Here's the drawing with two shaded views (mm, measured from the low corner). I have some questions. A direction names the side the tool comes from. Coordinates: 2 decimals unless noted, no trailing zeros. Loops run counter-clockwise (first coordinate to the right, second up) from the corner with the lowest first, then second, coordinate; pieces in that order, holes last. Notation, with made-up numbers: (74.5, 47.25) -> (133.5, 47.25) arc R20 cw to (133.5, 75.25) -> close; hole circle Ø5 at (44.25, -4.5). An arc over 180 degrees is marked (long way). Use CSV: the item, a comma, the result in double quotes. Start each with the question number.
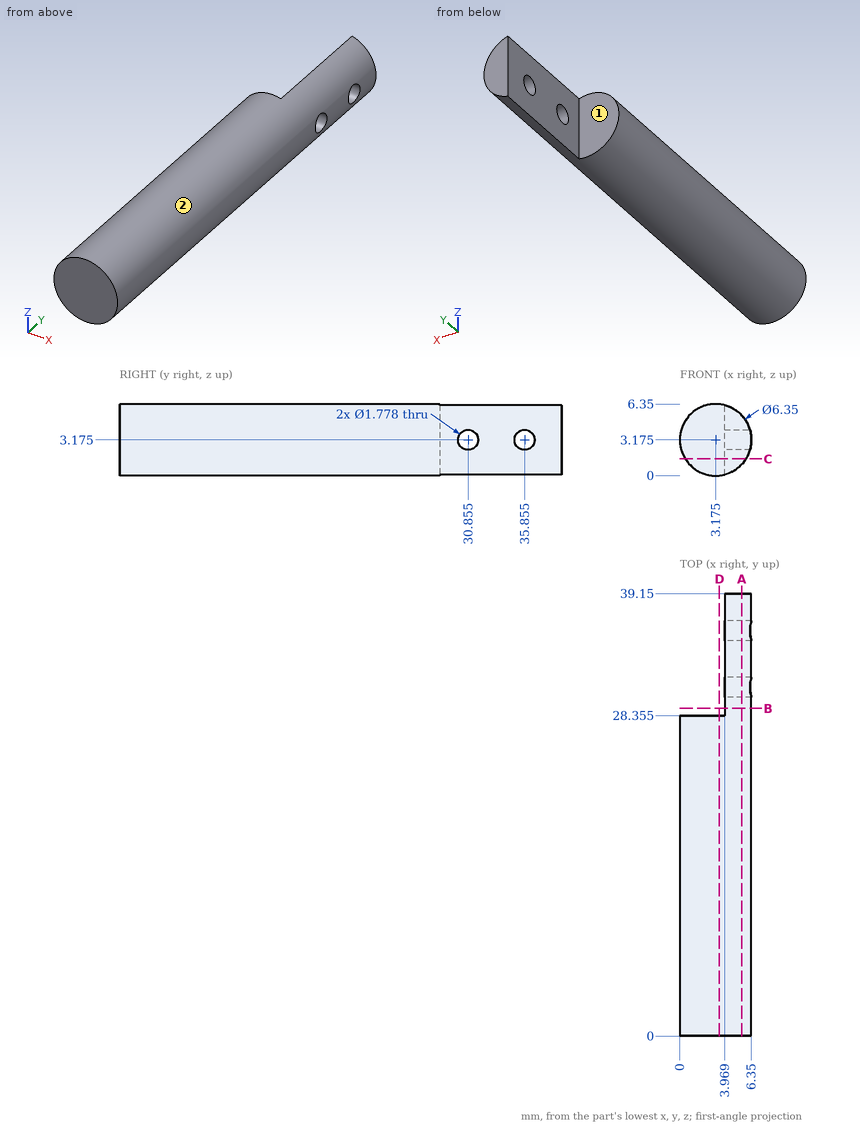
1) I want a section at D-D, the plane x = 3.5. Please give me the cut outline in (y, z) (3 decimals).
2) For P1, Ø1, axis at y = 17.5, z = 1.5, coming from the -X side; P2, Ø1, axis at x = 4, y = 31.5, coming from the -Z side; P3, Ø2, axis at x = 1.5, z = 3, coming from the +Y side (3 decimals), each with a flat end and sliding along its axis, tell me the tip position at first contact or that it passes through.
3) I want a section at A-A, the plane x = 5.5. Please give me the cut outline in (y, z) (3 decimals).
4) I want a section at B-B, the plane y = 29. Please give me the cut outline in (x, z) (3 decimals), plus the area to 3 significant figures.
5) I want a section at C-C, the plane z = 1.5. Please give me the cut outline in (x, y) (3 decimals).
6) Which directions (+Z, -Z, +X, -X, +Y, -Y) give clear straight access to the entire face, cutting with the end or side of a thin tool? Please do the marked faces 1 and 2.
7) Please list where these lines run through material, in increasing order: L1, parallel to Y at x = 6, z = 3.75; L2, parallel to Y at x = 4.5, z = 3.5; L3, parallel to Y at x = 1.5, z = 0.75 (3 decimals). Write a range as [from, to].
Return value:
1,outline,"(0, 0.017) -> (28.355, 0.017) -> (28.355, 6.333) -> (0, 6.333) -> close"
2,P1,"stops at x = 0.23"
2,P2,"stops at z = 0.1"
2,P3,"stops at y = 28.355"
3,outline,"(0, 1.013) -> (39.15, 1.013) -> (39.15, 5.337) -> (0, 5.337) -> close; hole circle Ø1.778 at (30.855, 3.175); hole circle Ø1.778 at (35.855, 3.175)"
4,outline,"(3.969, 0.101) arc R3.175 ccw to (3.969, 6.249) -> close"
4,area,"10.8 mm²"
5,outline,"(0.478, 0) -> (5.872, 0) -> (5.872, 39.15) -> (3.969, 39.15) -> (3.969, 28.355) -> (0.478, 28.355) -> close"
6,face 1,"+Z, -Z, -X, +Y"
6,face 2,"+Y, -Y"
7,L1,"y = [0, 30.18], [31.53, 35.18], [36.53, 39.15]"
7,L2,"y = [0, 30.03], [31.68, 35.03], [36.68, 39.15]"
7,L3,"y = [0, 28.355]"
